For this review, use the dimensioned drawing (mm, ordinates from the lowest corner) and the shaded views. A direction names the side the tool comes from. Round coordinates to 2 decimals unless told otherwise and drop trailing zeros. Loops run counter-clockwise (first coordinate to the right, second up) from the corner with the lowest first, then second, coordinate; pieces in that order, holes last. Notation, with made-up numbers: (24, -16) -> (39, -16) arc R24 ccw to (39, -6) -> close; hole circle Ø1 at (18, 23.25). An arc over 180 degrees is marked (long way). Write each question's results on one line, items separated by ' | '.
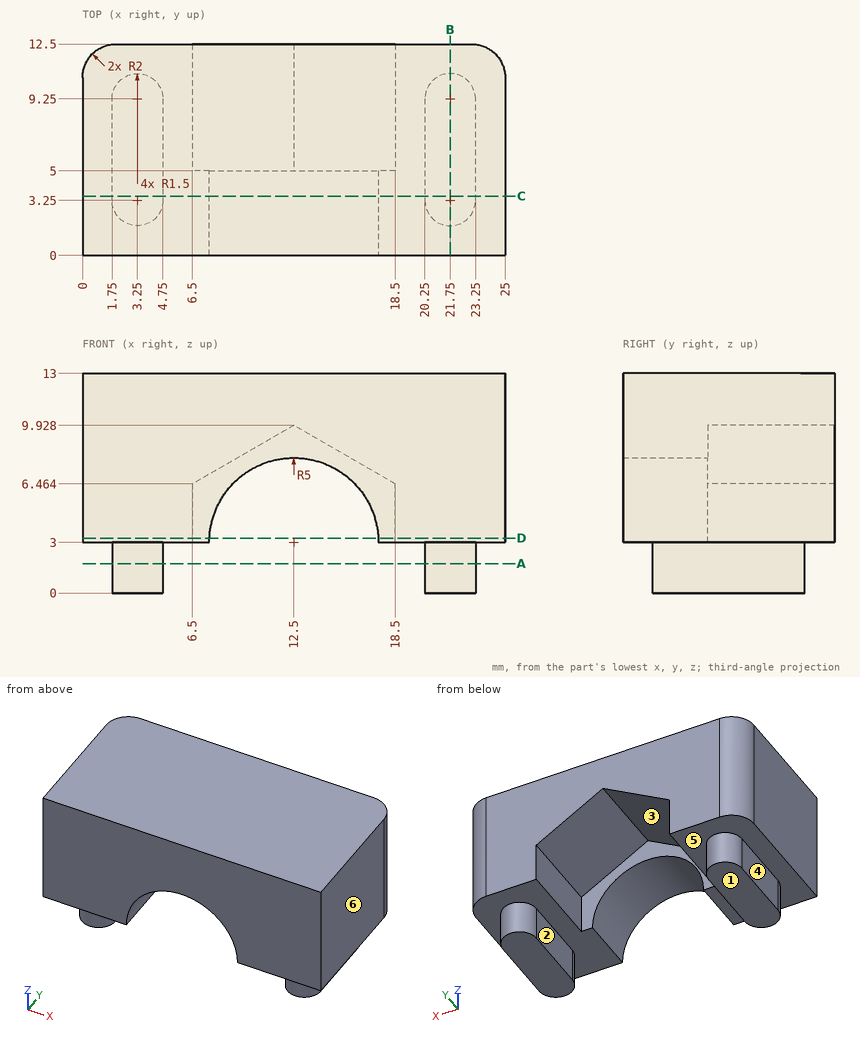
1. Draft analysis for pull direction X (two halves, no side actions). For the marked faces 4, 5 and 6, state which applies: released by +X, released by -X, zero draft, split by the parting line, or undercut.
Values found:
face 4: released by -X | face 5: undercut | face 6: released by +X
2. Tool access review of the marked faces 1, 2 and 3: name each direction out of +Z, -Z, +X, -X, +Y, -Y from which nothing blocks a thin tool from reaching the whole face with its end or side.
Values found:
face 1: -Z, +X, -X, +Y, -Y | face 2: -Z, +Y, -Y | face 3: -Z, +Y
3. Consider section A-A (z = 1.75). State the section outline as (x, y) points.
Values found:
outline: (1.75, 3.25) arc R1.5 ccw to (4.75, 3.25) -> (4.75, 9.25) arc R1.5 ccw to (1.75, 9.25) -> close; (20.25, 3.25) arc R1.5 ccw to (23.25, 3.25) -> (23.25, 9.25) arc R1.5 ccw to (20.25, 9.25) -> close
4. To check wall thickness, follow probe 1 along Z at (x, y) = (21.5, 11); probe 2 along X at (y, z) = (7, 6); probe 3 along X at (y, z) = (4.5, 0.5). State the ranges of each line that lie inside material, in increasing order.
Values found:
probe 1: z = 3 to 13 | probe 2: x = 0 to 6.5, 18.5 to 25 | probe 3: x = 1.75 to 4.75, 20.25 to 23.25
5. For pin 1 (1.5 mm diameter, centred on y = 5.5, z = 2, fed in from -X); pin 2 (3.5 mm diameter, centred on x = 10.5, z = 7.5, fed in from +Y); pin 3 (1.5 mm diameter, centred on x = 7.5, z = 2.5, fed in from +Y); pin 4 (3.5 mm diameter, centred on y = 5.5, z = 1, fed in from +X), all flat-tipped, find the tip position at first contact; note any pin that passes through.
Values found:
pin 1: stops at x = 1.75 | pin 2: stops at y = 12.5 | pin 3: stops at y = 5 | pin 4: stops at x = 23.25
6. Consider section B-B (x = 21.75). State the section outline as (y, z) points.
Values found:
outline: (0, 3) -> (1.75, 3) -> (1.75, 0) -> (10.75, 0) -> (10.75, 3) -> (12.5, 3) -> (12.5, 13) -> (0, 13) -> close
7. Consider section C-C (y = 3.5). State the section outline as (x, z) points.
Values found:
outline: (0, 3) -> (1.75, 3) -> (1.75, 0) -> (4.75, 0) -> (4.75, 3) -> (7.5, 3) arc R5 cw to (17.5, 3) -> (20.25, 3) -> (20.25, 0) -> (23.25, 0) -> (23.25, 3) -> (25, 3) -> (25, 13) -> (0, 13) -> close
8. Consider section D-D (z = 3.25). State the section outline as (x, y) points.
Values found:
outline: (0, 0) -> (7.51, 0) -> (7.51, 5) -> (6.5, 5) -> (6.5, 12.5) -> (2, 12.5) arc R2 ccw to (0, 10.5) -> close; (17.49, 0) -> (25, 0) -> (25, 10.5) arc R2 ccw to (23, 12.5) -> (18.5, 12.5) -> (18.5, 5) -> (17.49, 5) -> close
